from build123d import *

# Parameters (mm, degrees)
SKETCH1_W           = 120
SKETCH1_H           = 60
SKETCH1_R           = 4.5
BOSS_EXTRUDE1_DEPTH = 15
SKETCH2_R           = 20
SKETCH2_R_2         = 10
BOSS_EXTRUDE2_DEPTH = 60
BOSS_EXTRUDE3_DEPTH = 10
BOSS_EXTRUDE4_START = 3
SKETCH11_R          = 14
SKETCH11_R_2        = 4.5
BOSS_EXTRUDE4_DEPTH = 3
RIB1_REACH          = 126.599
SKETCH13_WALL_W     = 322.54976404
SKETCH13_WALL_H     = 8
FILLET1_R           = 2


with BuildPart() as part:
    # Sketch1 → Boss-Extrude1 (new body)
    with BuildSketch(Plane(origin=(0, 0, 0), x_dir=(1, 0, 0), z_dir=(0, 1, 0))):
        Rectangle(SKETCH1_W, SKETCH1_H)
        with Locations(Location((-35, 0, 0), (0, 0, 270))):
            Circle(SKETCH1_R, mode=Mode.SUBTRACT)
        with Locations(Location((35, 0, 0), (0, 0, 270))):
            Circle(SKETCH1_R, mode=Mode.SUBTRACT)
    extrude(amount=-BOSS_EXTRUDE1_DEPTH)



with BuildPart() as body_2:
    # Sketch2 → Boss-Extrude2 (new body)
    with BuildSketch(Plane.XY.offset(30)):
        with Locations((0, 85)):
            Circle(SKETCH2_R)
        with Locations((0, 85)):
            Circle(SKETCH2_R_2, mode=Mode.SUBTRACT)
    extrude(amount=-BOSS_EXTRUDE2_DEPTH)


with BuildPart() as part_1:
    add(part.part)

    add(body_2.part)  # Boss-Extrude3 merges body 2
    # Sketch3 → Boss-Extrude3 (add)
    with BuildSketch(Plane.XY.offset(30)):
        with BuildLine():
            Line((-60, 0), (-18.251723952, 93.177687496))
            ThreePointArc((-18.251723952, 93.177687496), (0, 65), (18.251723952, 93.177687496))
            Line((18.251723952, 93.177687496), (60, 0))
            Line((60, 0), (-60, 0))
        make_face()
    extrude(amount=-BOSS_EXTRUDE3_DEPTH)

    # Sketch11 → Boss-Extrude4 (add)
    # profile 1 of 2: a face of its own
    with BuildSketch(Plane(origin=(0, 0, 0), x_dir=(1, 0, 0), z_dir=(0, 1, 0)).offset(BOSS_EXTRUDE4_START)):
        with Locations(Location((-35, 0, 0), (0, 0, 270))):
            Circle(SKETCH11_R)
        with Locations(Location((-35, 0, 0), (0, 0, 270))):
            Circle(SKETCH11_R_2, mode=Mode.SUBTRACT)
    # profile 2 of 2: a face of its own
    with BuildSketch(Plane(origin=(0, 0, 0), x_dir=(1, 0, 0), z_dir=(0, 1, 0)).offset(BOSS_EXTRUDE4_START)):
        with Locations(Location((35, 0, 0), (0, 0, 270))):
            Circle(SKETCH11_R)
        with Locations(Location((35, 0, 0), (0, 0, 270))):
            Circle(SKETCH11_R_2, mode=Mode.SUBTRACT)
    extrude(amount=-BOSS_EXTRUDE4_DEPTH)

    # Sketch13 wall → Rib1 (add, up to next)
    with BuildSketch(Plane(origin=(0, 32.5, -14.713701713), x_dir=(0, 0.910988719631, 0.41243127028), z_dir=(0, -0.41243127028, 0.910988719631)), mode=Mode.PRIVATE) as rib1_sk1:
        Rectangle(SKETCH13_WALL_W, SKETCH13_WALL_H)
    rib1_tool1 = extrude(rib1_sk1.sketch, amount=RIB1_REACH, mode=Mode.PRIVATE) - part_1.part
    add(rib1_tool1.solids().sort_by_distance((0, 32.5, -14.713701713))[0])

    # Fillet1
    fillet1_edges = [part_1.edges().sort_by_distance(p)[0] for p in [
        (0, 65, -1e-09),
    ]]
    fillet(fillet1_edges, radius=FILLET1_R)


solid = part_1.part
Input: part model. Units: mm. Frame: model coordinates. A direction names the side the tool comes from. Coordinates: 2 decimals unless noted, no trailing zeros. Write each loop counter-clockwise with the first axis right and the second up, starting at its lowest first coordinate (ties: lowest second). Pieces come first, ordered by that corner, then holes. Notation, with made-up numbers: M 67,27 L 99,27 A20 cw 99,46 Z; hole C 54,40 d5. An arc over 180 degrees is marked long. Answer as a JSON object with one key per item and string values. Group by question number.
(1) Section C-C on z = 12.5. Output: boundary loops of the cut face in (x, y), plus the area to 3 significant figures.
(2) Section A-A on z = -25.5. Output: boundary loops of the cut face in (x, y).
(3) Section B-B on x = -35. Output: boundary loops of the cut face in (y, z), plus the area to 3 significant figures.
(4) Section D-D on y = 85. Output: boundary loops of the cut face in (x, z), plus the area to 3 significant figures.
(5) Mould query, pull axis Y, two halves, no side actions, for faces 1 (the face through (38.3, 3, -3.3)), 2 (the face through (-4, 30, 1)), 3 (the face through (4, 30, 1)), 4 (the face through (-1, -15, 0)). Classes: pulls with the +Y half, pulls with the -Y half, needs draft (parallel to the pull), parting line crosses it, or undercut.
(6) Ray query, line 1 along X through (y, z) = (-2.5, 0); line 2 along Y through (x, z) = (0, 14); line 3 along Y through (x, z) = (-4.5, -25). Return the intervals inside material, ascending. Write a range as [from, to].
(7) Contact query for flat-ended pins moving along their axis: P1, Ø14.5, axis at x = -35, z = 0, coming from the +Y side; P2, Ø3, axis at y = 46, z = 3.5, coming from the -X side; P3, Ø17, axis at x = -19.5, y = 49.5, coming from the -Z side. Output: stop coordinate, or through.
(8) Set-up query: faces 5 (the face through (-0.06, 30.83, -15.47)), 6 (the face through (21.33, 1.52, -3.03)), 7 (the face through (-2.6, 104.83, -6.25)), 8 (the face through (-31.7, 3, -3.3)), 9 (the face through (-39.418, 45.937, 25.07)). Return all of +Z, -Z, +X, -X, +Y, -Y with unobstructed straight access to the full face (end or side cutting, diameter ignored); none if empty.
Result set:
{
 "1": {"outline": "M -60,-15 L 60,-15 L 60,0 L 41.3,0 L 41.3,3 L 28.7,3 L 28.7,0 L 4,0 L 4,65.4 A20 ccw long -4,65.4 L -4,0 L -28.7,0 L -28.7,3 L -41.3,3 L -41.3,0 L -60,0 Z; hole C 0,85 d20", "area": "3,340 mm2"},
 "2": {"outline": "M -60,-15 L 60,-15 L 60,0 L 4,0 L 4,8.67 L -4,8.67 L -4,0 L -60,0 Z; C 0,85 d40; hole C 0,85 d20"},
 "3": {"outline": "M -15,-30 L 0,-30 L 0,-14 L 3,-14 L 3,-4.5 L -15,-4.5 Z; M -15,4.5 L 3,4.5 L 3,14 L 0,14 L 0,20 L 55.8,20 L 55.8,30 L -15,30 Z", "area": "1,380 mm2"},
 "4": {"outline": "M -21.92,20 L -20,20 L -20,-30 L -10,-30 L -10,30 L -21.92,30 Z; M 10,-30 L 20,-30 L 20,20 L 21.92,20 L 21.92,30 L 10,30 Z", "area": "1,240 mm2"},
 "5": {"face 1": "pulls with the +Y half", "face 2": "undercut", "face 3": "undercut", "face 4": "pulls with the -Y half"},
 "6": {"line 1": "x = [-60, -39.5], [-30.5, 30.5], [39.5, 60]", "line 2": "y = [-15, 75], [95, 105]", "line 3": "y = [-15, 0], [65.51, 76.07], [93.93, 104.49]"},
 "7": {"P1": "stops at y = 3", "P2": "stops at x = -4", "P3": "stops at z = 20"},
 "8": {"face 5": "-Z, +X, -X", "face 6": "+Y", "face 7": "-Z", "face 8": "-Z, -X, +Y", "face 9": "+Z, -Z, -X, +Y"}
}
